Work out the finished part from the listing and answer in its coordinate system (mm). Face numbers are marked on the shaded views. Give positions to 0.01 mm unless a question says otherwise; leave off trailing zeros. Loops run counter-clockwise (first coordinate to the right, second up) from the corner with the lowest first, then second, coordinate; pieces in that order, holes last. Notation, with made-up numbers: (27, 81) -> (79, 81) arc R15 cw to (79, 92) -> close; hole circle Ø8 at (7.5, 56.5). An arc over 180 degrees is marked (long way). Answer as CSV lines item,"result". Start each with the question number.
1. Find section D-D, the plane y = 45.4. Give the vertices of the cut face in (x, z), and give its area (3 significant figures).
2. Determine the mould class of the marked faces 1 and 2 for opening direction X: +X half, -X half, draft (parallel to the pull), parting line (faces both ways), or undercut.
3. A flat-ended cylindrical pin translates along its axis: pin 1 Ø3 at (x, y) = (38.5, 44) entering from +Z. Find the tip coordinate at first contact, or state that the pin passes through.
4. Find section C-C, the plane x = 28. Give the vertices of the cut face in (y, z).
5. Find section B-B, the plane x = 10. Give the vertices of the cut face in (y, z).
6. Find section A-A, the plane y = 38.5. Give the vertices of the cut face in (x, z).
7. Find the intervals of material crossed by line 1 along Y through (x, z) = (10, 0.65); line 2 along X through (y, z) = (38.25, 0.75); line 3 along Z through (x, y) = (6, 34.5), in increasing order.
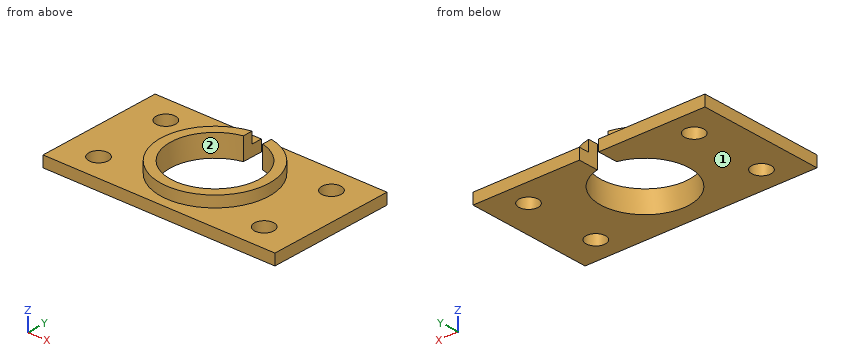
from build123d import *

# Parameters (mm, degrees)
SKETCH_2_W               = 42
SKETCH_2_H               = 23
EXTRUDE_1_DEPTH          = 2
SKETCH_3_R               = 9.75
EXTRUDE_2_DEPTH          = 2
SKETCH_4_R               = 8
CUT_EXTRUDE_1_DEPTH      = 69.058798109
CUT_EXTRUDE_2_DEPTH      = 69.058798109
CUT_EXTRUDE_2_DEPTH_BACK = 69.058798109
SKETCH_5_R               = 1.75
CUT_EXTRUDE_4_REACH      = 70.059
SKETCH_7_W               = 3.5
SKETCH_7_H               = 14.451393072


with BuildPart() as part:
    # 草图2 → 凸台-拉伸1 (new body)
    with BuildSketch(Plane.XY):
        with Locations((25, 38.5)):
            Rectangle(SKETCH_2_W, SKETCH_2_H)
    extrude(amount=EXTRUDE_1_DEPTH)

    # 草图3 → 凸台-拉伸2 (add)
    with BuildSketch(Plane.XY.offset(2)):
        with Locations((25, 38.5)):
            Circle(SKETCH_3_R)
    extrude(amount=EXTRUDE_2_DEPTH)

    # 草图4 → 切除-拉伸1 (cut, through all)
    with BuildSketch(Plane.XY.offset(4)):
        with Locations((25, 38.5)):
            Circle(SKETCH_4_R)
    extrude(amount=-CUT_EXTRUDE_1_DEPTH, mode=Mode.SUBTRACT)

    # 草图5 → 切除-拉伸2 (cut, two sides: drawn at the far end of the back side and taken through both)
    with BuildSketch(Plane(origin=(0, 0, 0), x_dir=(-1, 0, 0), z_dir=(0, 0, -1)).offset(-CUT_EXTRUDE_2_DEPTH_BACK)):
        with Locations(Location((-40, 45.4, 0), (0, 0, 180))):
            Circle(SKETCH_5_R)
        with Locations(Location((-40, 31.6, 0), (0, 0, 180))):
            Circle(SKETCH_5_R)
        with Locations(Location((-10, 31.6, 0), (0, 0, 180))):
            Circle(SKETCH_5_R)
        with Locations(Location((-10, 45.4, 0), (0, 0, 180))):
            Circle(SKETCH_5_R)
    extrude(amount=CUT_EXTRUDE_2_DEPTH + CUT_EXTRUDE_2_DEPTH_BACK, mode=Mode.SUBTRACT)

    # 草图7 → 切除-拉伸4 (cut, up to next)
    with BuildSketch(Plane(origin=(0, 0, 0), x_dir=(-1, 0, 0), z_dir=(0, 0, -1)), mode=Mode.PRIVATE) as cut_extrude_4_sk1:
        with Locations((-25, 46.889165471)):
            Rectangle(SKETCH_7_W, SKETCH_7_H)
    cut_extrude_4_tool1 = extrude(cut_extrude_4_sk1.sketch, amount=-CUT_EXTRUDE_4_REACH, mode=Mode.PRIVATE) & part.part
    add(cut_extrude_4_tool1.solids().sort_by_distance((25, 46.889165, 0))[0], mode=Mode.SUBTRACT)


solid = part.part
Resolved:
1,outline,"(4, 0) -> (8.25, 0) -> (8.25, 2) -> (4, 2) -> close; (11.75, 0) -> (20.95, 0) -> (20.95, 4) -> (18.11, 4) -> (18.11, 2) -> (11.75, 2) -> close; (29.05, 0) -> (38.25, 0) -> (38.25, 2) -> (31.89, 2) -> (31.89, 4) -> (29.05, 4) -> close; (41.75, 0) -> (46, 0) -> (46, 2) -> (41.75, 2) -> close"
1,area,"65.2 mm^2"
2,face 1,"draft"
2,face 2,"undercut"
3,pin 1,"stops at z = 2"
4,outline,"(27, 0) -> (31.08, 0) -> (31.08, 4) -> (29.22, 4) -> (29.22, 2) -> (27, 2) -> close; (45.92, 0) -> (50, 0) -> (50, 2) -> (47.78, 2) -> (47.78, 4) -> (45.92, 4) -> close"
5,outline,"(27, 0) -> (29.85, 0) -> (29.85, 2) -> (27, 2) -> close; (33.35, 0) -> (43.65, 0) -> (43.65, 2) -> (33.35, 2) -> close; (47.15, 0) -> (50, 0) -> (50, 2) -> (47.15, 2) -> close"
6,outline,"(4, 0) -> (17, 0) -> (17, 4) -> (15.25, 4) -> (15.25, 2) -> (4, 2) -> close; (33, 0) -> (46, 0) -> (46, 2) -> (34.75, 2) -> (34.75, 4) -> (33, 4) -> close"
7,line 1,"y = 27 to 29.85, 33.35 to 43.65, 47.15 to 50"
7,line 2,"x = 4 to 17, 33 to 46"
7,line 3,"z = 0 to 2"
